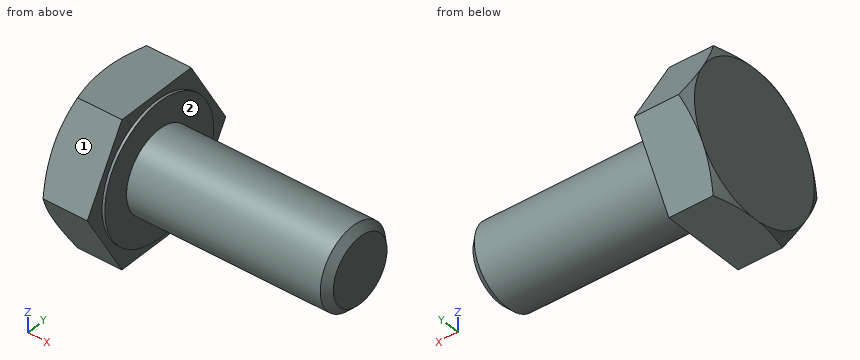
Autodesk Inventor part; units mm, degrees
ref_plane "Work Plane1" through (1.525, 0, 0) normal (0, 0, 1) x (1, 0, 0)
ref_plane "YZ Plane" through (0, 0, 0) normal (1, 0, 0) x (0, 1, 0)
ref_plane "XZ Plane" through (0, 0, 0) normal (0, 1, 0) x (-1, 0, 0)
sketch "Sketch1" plane through (0, 0, 0) normal (0, 0, 1) x (1, 0, 0)
  line L0 (0, 10) -> (0, 6)
  line L1 (9, 6) -> (30, 6)
  line L2 (30, 6) -> (30, 0)
  line L3 (30, 0) -> (-0.4001, 0)
  line L4 (-6.4801, 0) -> (36.08, 0)
  line L5 (-0.4001, 0) -> (-0.4001, 10)
  line L6 (-0.4001, 10) -> (0, 10)
  line L7 (9, 6) -> (7.9264, 6)
  line L8 (7.9264, 6) -> (0, 6)
  line L9 (0, -2) -> (0, 12)
  dimension "d0" = 30
  dimension "d1" = 21
  dimension "d2" = 12
  dimension "d9" = 0.4001
  dimension "d10" = 20
  dimension "d13" = 1.0736
  dimension "d14" = 12
revolve "Body" add sketch "Sketch1" angle 360 about axis through (30, 0, 0) along (-1, 0, 0)
sketch "Sketch2" plane through (-0.4001, 0, 0) normal (-1, 0, 0) x (0, 0, 1)
  line L0 (0, 12.7017) -> (11, 6.3509)
  line L1 (11, 6.3509) -> (11, -6.3509)
  line L2 (11, -6.3509) -> (0, -12.7017)
  line L3 (0, -12.7017) -> (-11, -6.3509)
  line L4 (-11, -6.3509) -> (-11, 6.3509)
  line L5 (-11, 6.3509) -> (0, 12.7017)
  point P0 (0, 0)
  point P1 (0, 0)
  dimension "d11" = 22
extrude "Head" add sketch "Sketch2" along normal blind 7.6
sketch "Sketch4" plane through (0, 0, 0) normal (0, 0, 1) x (1, 0, 0)
  line L0 (-8.0001, 11) -> (-8.0001, 12.7017)
  line L1 (-8.0001, 12.7017) -> (-7.0176, 12.7017)
  line L2 (-7.0176, 12.7017) -> (-8.0001, 11)
  line L3 (-9.5201, 0) -> (1.1199, 0)
  line L4 (-0.4001, 12.7017) -> (-8.0001, 12.7017)
  line L5 (-8.0001, 6.3509) -> (-8.0001, 12.7017)
  dimension "d5" = 30
  dimension "d19" = 22
revolve "Chamfer1" cut sketch "Sketch4" angle 360 about axis through (-10, 0, 0) along (1, 0, 0)
thread "Thread"
chamfer "Chamfer2" distance 1.0735 distance2 1.0736 1 edges at (30, -6, 0) measured on face at (30, -2.3028, 0.7984)
ref_plane "Work Plane1" through (1.525, 0, 0) normal (0, 0, 1) x (1, 0, 0)
equation "\"d0\" = NLG"
equation "\"d1\" = GEL"
equation "\"d2\" = GD"
equation "\"d10\" = SD2"
equation "\"d14\" = BDM"
equation "\"d11\" = SW"
equation "\"d3\" = KOH - SD"
equation "\"d5\" = ANG1"
equation "\"d19\" = SW0"
equation "\"d15\" = GEL"
equation "\"d6\" = -0.5 * SPD + 0.5 * GD"
equation "\"NLG\" = 30"
equation "\"GD\" = NND"
equation "\"BDM\" = NND"
equation "\"KOH\" = 8"
equation "\"GEL\" = 21"
equation "\"SW\" = 22"
equation "\"SW0\" = SW"
equation "\"SPD\" = NND - 1.2269 * PTC"
equation "\"SD2\" = SDH"
equation "\"SD\" = 0.4"
equation "\"ANG1\" = 30deg"
equation "\"GAL\" = 0.61345 * PTC"
equation "\"GUL\" = 0.61345 * PTC"
equation "\"RR\" = 1.2"
equation "\"WFT\" = 0.4"
equation "\"GD1\" = THREADDIA - 1.2269 * PTC"
equation "\"THREADDIA\" = 12"
equation "\"TOA\" = 30deg"
equation "\"FAWI\" = 45deg"
equation "\"PTC\" = 1.75"
equation "\"NND\" = 12"
equation "\"E0\" = 1.155 * SW"
equation "\"K1\" = 5.28"
properties part number "DIN 6914 - M12 x 30" material "Steel, Mild"
Input: part model. Units: mm. Frame: model coordinates. Face numbers are marked on the shaded views. A direction names the side the tool comes from. Round coordinates to 2 decimals unless told otherwise and drop trailing zeros. Write each loop counter-clockwise with the first axis right and the second up, starting at its lowest first coordinate (ties: lowest second). Pieces come first, ordered by that corner, then holes. Notation, with made-up numbers: (28.25, 62.25) -> (51.25, 62.25) arc R22 ccw to (51.25, 92.25) -> close; hole circle Ø11 at (-3, 80.25). An arc over 180 degrees is marked (long way). Answer as CSV lines item,"result".
1. Reachability of the marked faces 1 and 2 from +Z, -Z, +X, -X, +Y, -Y: full face, straight path, thin tool, end or side. Return the list, or none.
Geometry says:
face 1,"+Z, +X, -X, -Y"
face 2,"+X"
2. Section B-B (x = 20). Return the cut outline in (y, z), plus the area to 3 significant figures.
Geometry says:
outline,"circle Ø12 at (0, 0)"
area,"113 mm^2"
3. Section A-A (x = -2). Return the cut outline in (y, z), plus the area to 3 significant figures.
Geometry says:
outline,"(-12.7, 0) -> (-6.35, -11) -> (6.35, -11) -> (12.7, 0) -> (6.35, 11) -> (-6.35, 11) -> close"
area,"419 mm^2"
4. Ray query, L1, parallel to X at y = 4.5, z = -9; L2, parallel to X at y = -4.25, z = 5.25; L3, parallel to Y at x = 19, z = -0.25. Return the intervals inside material, ascending. Write a range as [from, to].
Geometry says:
L1,"x = [-8, -0.4]"
L2,"x = [-8, 0]"
L3,"y = [-5.99, 5.99]"
5. Contact query for flat-ended pins moving along their axis: P1, Ø12, axis at x = 16.5, y = -8.5, coming from the -Z side; P2, Ø5, axis at y = -5, z = -6, coming from the +X side; P3, Ø1, axis at x = 11, z = -1.5, coming from the +Y side. Output: stop coordinate, or through.
Geometry says:
P1,"stops at z = -5.45"
P2,"stops at x = 29.62"
P3,"stops at y = 5.92"
